CAD build for the part. Positions are in the model's coordinates, mm. A direction names the side the tool comes from. Coordinates: 2 decimals unless noted, no trailing zeros. Loops run counter-clockwise (first coordinate to the right, second up) from the corner with the lowest first, then second, coordinate; pieces in that order, holes last.
1) Saw through at B-B, the plane y = 0. Write the cut outline in (x, z).
2) Two-plate mould, pull along X, no slides. Class faces 1 (the flat face through (-3.513, -5.972, -2.535)), 2 (the flat face through (0, -3, 14)), 3 (the flat face through (-6.928, 0, -3)): +X half, -X half, draft (parallel to the pull), parting line (faces both ways), or undercut.
3) Saw through at C-C, the plane z = 5.25. Write the cut outline in (x, y), and give its area (3 significant figures).
4) Saw through at A-A, the plane x = 12. Write the cut outline in (y, z), and give its area (3 significant figures).
5) Pin check, flat tips, straight feed: pin 1 Ø2.5 at (y, z) = (1.5, -2) entering from -X; pin 2 Ø6 at (x, y) = (0, 0) entering from -Z; pin 3 Ø1 at (x, z) = (-2.5, 2.5) entering from -Y. Stop position of each tip, or through.
6) Wall check: line 1 along Y through (x, z) = (0, 5); line 2 along Z through (x, y) = (6.25, 0); line 3 along Z through (x, y) = (10, 0). Give the ranges that are in metal, low to high.
7) Saw through at D-D, the plane y = -7. Write the cut outline in (x, z), and give its area (3 significant figures).
8) Which spindle directions (+Z, -Z, +X, -X, +Y, -Y) get a long thin tool onto all of the face, cutting with end or side? Do faces 4 (the cylindrical face through (-2.248, 0.099, 7.098)), 5 (the cylindrical face through (8.288, -0.303, 11.367)), 6 (the flat face through (-3.416, 6.028, -2.535)). Say none if no direction does.
Autodesk Inventor part; units mm, degrees
ref_plane "YZ Plane" through (0, 0, 0) normal (1, 0, 0) x (0, 1, 0)
ref_plane "XZ Plane" through (0, 0, 0) normal (0, 1, 0) x (-1, 0, 0)
ref_plane "XY Plane" through (0, 0, 0) normal (0, 0, 1) x (1, 0, 0)
sketch "Sketch1" plane through (0, 0, 0) normal (0, 0, 1) x (1, 0, 0)
  circle A0 centre (0, 0) radius 15
  dimension "d0" = 30
extrude "Extrusion1" add sketch "Sketch1" along normal blind 14
sketch "Sketch2" plane through (0, 0, 14) normal (0, 0, 1) x (1, 0, 0)
  circle A0 centre (0, 0) radius 2.25
  dimension "d3" = 4.5
extrude "Extrusion2" cut sketch "Sketch2" against normal blind 19
sketch "Sketch3" plane through (0, 0, 0) normal (0, 0, -1) x (-1, 0, 0)
  circle A0 centre (0, 0) radius 15
extrude "Extrusion3" add sketch "Sketch3" along normal blind 5
sketch "Sketch6" plane through (0, 0, -5) normal (0, 0, -1) x (-1, 0, 0)
  line L0 (0, -8) -> (-6.9282, -4)
  line L1 (-6.9282, -4) -> (-6.9282, 4)
  line L2 (-6.9282, 4) -> (0, 8)
  line L3 (0, 8) -> (6.9282, 4)
  line L4 (6.9282, 4) -> (6.9282, -4)
  line L5 (6.9282, -4) -> (0, -8)
  point P0 (0, 0)
  point P1 (0, 0)
  dimension "d15" = 16
extrude "Extrusion6" cut sketch "Sketch6" against normal blind 5
sketch "Sketch7" plane through (0, 0, 0) normal (1, 0, 0) x (0, 1, 0)
  circle A0 centre (0, 10) radius 1.4
  line L0 (15, 14) -> (-15, 14)
  point P0 (0, 0)
  dimension "d18" = 2.8
  dimension "d22" = 4
extrude "Extrusion7" cut sketch "Sketch7" along normal through all
properties part number "AA009" material "ABS Plastic"
Data:
1. outline: (-15, -5) - (-6.93, -5) - (-6.93, 0) - (-2.25, 0) - (-2.25, 14) - (-15, 14) - close; (2.25, 0) - (6.93, 0) - (6.93, -5) - (15, -5) - (15, 8.6) - (2.25, 8.6) - close; (2.25, 11.4) - (15, 11.4) - (15, 14) - (2.25, 14) - close
2. face 1: undercut
2. face 2: draft
2. face 3: undercut
3. outline: circle Ø30 at (0, 0); hole circle Ø4.5 at (0, 0)
3. area: 691 mm2
4. outline: (-9, -5) - (9, -5) - (9, 14) - (-9, 14) - close; hole circle Ø2.8 at (0, 10)
4. area: 336 mm2
5. pin 1: stops at x = -15
5. pin 2: stops at z = 0
5. pin 3: stops at y = -14.87
6. line 1: y = -15 to -2.25, 2.25 to 15
6. line 2: z = 0 to 8.6, 11.4 to 14
6. line 3: z = -5 to 8.6, 11.4 to 14
7. outline: (-13.27, -5) - (-1.73, -5) - (-1.73, 0) - (1.73, 0) - (1.73, -5) - (13.27, -5) - (13.27, 14) - (-13.27, 14) - close
7. area: 487 mm2
8. face 4: +Z, -Z
8. face 5: +X
8. face 6: -Z
